```python
from build123d import *

# Parameters (mm, degrees)
SKETCH1_W                      = 12.7
SKETCH1_H                      = 12.7
BOSS_EXTRUDE1_DEPTH            = 25.4
F_1_4_0_25_DIAMETER_HOLE1_D    = 6.35
SKETCH4_W                      = 1.27
SKETCH4_H                      = 7.62
CUT_EXTRUDE1_DEPTH             = 32.108519733
TAP_DRILL_FOR_10_32_TAP1_DEPTH = 18.986851973
F_6_CLEARANCE_HOLE1_D          = 3.7973
F_6_CLEARANCE_HOLE1_DEPTH      = 5.715
TAP_DRILL_FOR_6_32_TAP1_D      = 2.7051


# Read off the part's stored shape, not the designer's step: Tap Drill for #10-32 Tap1
with BuildPart() as part:
    # Sketch1 → Boss-Extrude1 (new body)
    with BuildSketch(Plane(origin=(0, 0, 0), x_dir=(1, 0, 0), z_dir=(0, 1, 0))):
        with Locations((6.35, 6.35)):
            Rectangle(SKETCH1_W, SKETCH1_H)
    extrude(amount=BOSS_EXTRUDE1_DEPTH)

    # 1/4 (0.25) Diameter Hole1 (through all)
    with Locations(Plane(origin=(12.7, 0, 0), x_dir=(0, 0, -1), z_dir=(1, 0, 0))):
        with Locations((6.35, 15.875)):
            Hole(F_1_4_0_25_DIAMETER_HOLE1_D / 2)

    # Sketch4 → Cut-Extrude1 (cut, through all)
    with BuildSketch(Plane(origin=(12.7, 0, 0), x_dir=(0, 0, -1), z_dir=(1, 0, 0))):
        with Locations((6.35, 21.59)):
            Rectangle(SKETCH4_W, SKETCH4_H)
    extrude(amount=-CUT_EXTRUDE1_DEPTH, mode=Mode.SUBTRACT)

    # Tap Drill for #10-32 Tap1 outline → Tap Drill for #10-32 Tap1 (cut)
    with BuildSketch(Plane(origin=(0, 0, 0), x_dir=(1, 0, 0), z_dir=(0, 1, 0))):
        with BuildLine():
            ThreePointArc((8.266858756, 5.715), (8.3693, 6.35), (8.266858756, 6.985))
            ThreePointArc((8.266858756, 6.985), (6.35, 8.3693), (4.433141244, 6.985))
            ThreePointArc((4.433141244, 6.985), (4.3307, 6.35), (4.433141244, 5.715))
            ThreePointArc((4.433141244, 5.715), (6.35, 4.3307), (8.266858756, 5.715))
        make_face()
    extrude(amount=TAP_DRILL_FOR_10_32_TAP1_DEPTH, mode=Mode.SUBTRACT)

    # #6 Clearance Hole1
    with Locations(Plane.XY):
        with Locations((6.35, 22.225)):
            Hole(F_6_CLEARANCE_HOLE1_D / 2, depth=F_6_CLEARANCE_HOLE1_DEPTH)

    # Tap Drill for #6-32 Tap1 (through all)
    with Locations(Plane.XY.offset(-6.985)):
        with Locations((6.35, 22.225)):
            Hole(TAP_DRILL_FOR_6_32_TAP1_D / 2)


solid = part.part
```
Build history of the part. All positions in model axes, mm. A direction names the side the tool comes from. Round coordinates to 2 decimals unless told otherwise and drop trailing zeros. Loops run counter-clockwise (first coordinate to the right, second up) from the corner with the lowest first, then second, coordinate; pieces in that order, holes last.
Item 1: Saw through at B-B (z = -6.35). List the corners of the cut face in (x, y), then the cut area to 3 significant figures.
Item 2: Saw through at A-A (x = 6.35). List the corners of the cut face in (y, z) (3 decimals).
Item 3: Which spindle directions (+Z, -Z, +X, -X, +Y, -Y) get a long thin tool onto all of the face, cutting with end or side? Do faces 1 (the face through (6.31, 18.72, -4.33)), 2 (the face through (6, 25.4, -3)), 3 (the face through (8, 22, -6.985)). Say none if no direction does.
Item 4: Saw through at D-D (z = -3.5). List the corners of the cut face in (x, y) (3 decimals), then the cut area to 3 significant figures.
Item 5: Two-plate mould, pull along Z, no slides. Class faces 4 (the face through (6, 18.987, -5)), 5 (the face through (6.597, 24.107, -2.898)), 6 (the face through (6.39, 18.72, -8.37)), 7 (the face through (6, 13, 0)): released by +Z, released by -Z, zero draft, split by the parting line, or undercut.
Item 6: Drill centre lines: line 1 along Y through (x, z) = (6.35, -10.85); line 2 along Y through (x, z) = (6.35, -1.8); line 3 along Z through (x, y) = (4.5, 20) (3 decimals). Where is each one in solid material? Low to high.
Item 7: Saw through at C-C (y = 12.25). List the corners of the cut face in (x, z) (3 decimals).
Worked answers:
1. outline: (0, 0) - (4.33, 0) - (4.33, 12.7) - (0, 12.7) - close; (8.37, 0) - (12.7, 0) - (12.7, 12.7) - (8.37, 12.7) - close
1. area: 110 mm2
2. outline: (0, -12.7) - (20.872, -12.7) - (20.872, -6.985) - (18.987, -6.985) - (18.987, -8.369) - (18.325, -8.369) arc R3.175 cw to (13.425, -8.369) - (0, -8.369) - close; (0, -4.331) - (13.425, -4.331) arc R3.175 cw to (18.325, -4.331) - (18.987, -4.331) - (18.987, -5.715) - (20.326, -5.715) - (20.326, 0) - (0, 0) - close; (23.578, -12.7) - (25.4, -12.7) - (25.4, -6.985) - (23.578, -6.985) - close; (24.124, -5.715) - (25.4, -5.715) - (25.4, 0) - (24.124, 0) - close
3. face 1: -Y
3. face 2: +Z, -Z, +X, -X, +Y
3. face 3: +X, -X, +Y
4. outline: (0, 0) - (12.7, 0) - (12.7, 14.476) - (0, 14.476) - close; (0, 17.274) - (12.7, 17.274) - (12.7, 25.4) - (0, 25.4) - close; hole circle Ø3.797 at (6.35, 22.225)
4. area: 276 mm2
5. face 4: undercut
5. face 5: zero draft
5. face 6: undercut
5. face 7: released by +Z
6. line 1: y = 0 to 20.87, 23.58 to 25.4
6. line 2: y = 0 to 20.33, 24.12 to 25.4
6. line 3: z = -12.7 to -6.985, -5.715 to 0
7. outline: (0, -12.7) - (12.7, -12.7) - (12.7, 0) - (0, 0) - close; hole circle Ø4.039 at (6.35, -6.35)
